The model under review builds one solid part; all positions refer to its coordinate system, in mm. Coordinates: 2 decimals unless noted, no trailing zeros. Order: outer loops, then holes, each group sorted by start corner. A loop starts at its lowest first (then second) coordinate and runs counter-clockwise, first axis right, second up. Notation, with made-up numbers: M -4.75,15.5 L 22.25,15.5 A34 ccw 22.25,48.5 Z; hole C 38,24.5 d2. An arc over 180 degrees is marked long. Answer as CSV lines item,"result". Start each with the question number.
Q1. Consider section A-A on x = 0. State how many separate pieces and enclosed holes the cut face has, and give its area (3 significant figures).
Q2. Wall thickness on L1, parallel to Z at x = 0, y = 1.75 (1 decimal); L2, parallel to Z at x = 10, y = 5.5; L3, parallel to Z at x = -1, y = 2.75: over which ranges is each line inside the solid? List them lowest first. Write a range as [from, to].
Q3. Consider section B-B on z = 81. Write out the cut boundary in (x, y), and give its area (3 significant figures).
Q4. For P1, Ø2, axis at x = 7, y = 5.5, coming from the -Z side; P2, Ø1, axis at y = 3, z = 38, coming from the -X side, all flat-tipped, find the tip position at first contact; note any pin that passes through.
Q5. Consider section C-C on x = -9.5. Write out the cut boundary in (y, z).
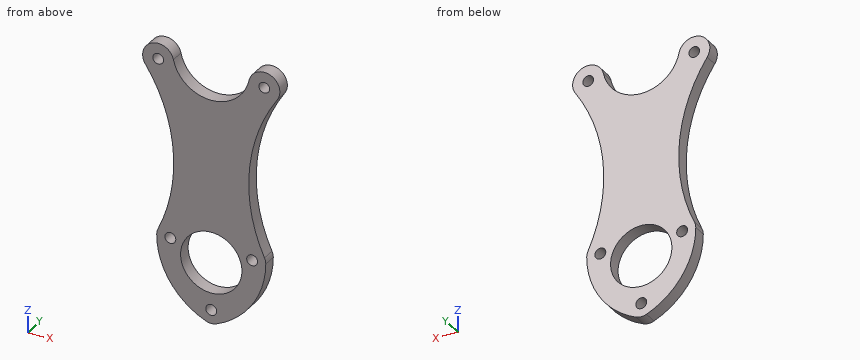
Autodesk Inventor part; units mm, degrees
ref_plane "YZ Plane" through (0, 0, 0) normal (1, 0, 0) x (0, 1, 0)
ref_plane "XZ Plane" through (0, 0, 0) normal (0, 1, 0) x (-1, 0, 0)
ref_plane "XY Plane" through (0, 0, 0) normal (0, 0, 1) x (1, 0, 0)
sketch "Sketch1" plane through (0, 0, 0) normal (0, 1, 0) x (-1, 0, 0)
  circle A0 centre (0, 0) radius 14.2875
  line L0 (143.7805, 15.875) -> (-143.7805, 15.875) construction
  line L1 (0, 0) -> (0, 15.875) construction
  line L2 (0, 15.875) -> (0, 88.9254) construction
  line L3 (24.6957, 88.9254) -> (-24.6957, 88.9254) construction
  line L4 (0, 113.6211) -> (0, 64.2297) construction
  circle A1 centre (24.6957, 88.9254) radius 2.4892
  circle A2 centre (-24.6957, 88.9254) radius 2.4892
  circle A3 centre (0, 64.2297) radius 2.4892 construction
  circle A4 centre (0, 113.6211) radius 2.4892 construction
  circle A5 centre (0, 0) radius 50.8 construction
  line L5 (143.7805, -34.925) -> (-143.7805, -34.925) construction
  line L6 (0, 0) -> (0, -34.925) construction
  circle A6 centre (19.05, 6.35) radius 2.54
  circle A7 centre (-19.05, 6.35) radius 2.54
  circle A8 centre (0, -22.225) radius 2.54
  line L7 (19.05, 6.35) -> (-19.05, 6.35) construction
  arc A9 (-2.4454, -28.0852) -> (2.4454, -28.0852) centre (0, -22.225) ccw
  arc A10 (-24.7931, 9.059) -> (-25.4, 6.3466) centre (-19.05, 6.35) ccw
  arc A11 (25.4, 6.3466) -> (24.7931, 9.059) centre (19.05, 6.35) ccw
  arc A12 (30.6963, 84.8535) -> (24.7931, 9.059) centre (94.1678, 41.783) ccw
  arc A13 (-24.7931, 9.059) -> (-30.6963, 84.8535) centre (-94.1678, 41.783) ccw
  arc A14 (2.4454, -28.0852) -> (25.4, 6.3466) centre (-11.9308, 6.3664) ccw
  arc A15 (-25.4, 6.3466) -> (-2.4454, -28.0852) centre (11.9308, 6.3664) ccw
  line L8 (12.3733, -7.1438) -> (20.6222, -11.9063) construction
  arc A16 (-17.6059, 90.4493) -> (-30.6963, 84.8535) centre (-24.6957, 88.9254) ccw
  arc A17 (30.6963, 84.8535) -> (17.6059, 90.4493) centre (24.6957, 88.9254) ccw
  arc A18 (-17.6059, 90.4493) -> (17.6059, 90.4493) centre (0, 94.2334) ccw
  line L9 (-17.4625, 41.783) -> (17.4625, 41.783) construction
  circle A19 centre (0, 88.9254) radius 12.7 construction
  point P0 (0, 6.35)
  dimension "d0" = 28.575
  dimension "d1" = 15.875
  dimension "d3" = 4.9784
  dimension "d4" = 88.9254
  dimension "d5" = 101.6
  dimension "d7" = 50.8
  dimension "d8" = 5.08
  dimension "d9" = 9.525
  dimension "d10" = 38.1
  dimension "d12" = 6.35
  dimension "d18" = 28.575
  dimension "d19" = 9.525
  dimension "d20" = 60
  dimension "d23" = 34.925
  dimension "d25" = 4.7625
  dimension "d26" = 34.925
  dimension "d27" = 25.4
extrude "Extrusion1" add sketch "Sketch1" along normal blind 6.35
properties material "Aluminum 6061"
Evaluation:
1,separate pieces,"3"
1,enclosed holes,"0"
1,area,"452 mm²"
2,L1,"z = [-28.6, -24.8], [-19.7, -14.3], [14.3, 76.2]"
2,L2,"z = [-23.84, -10.2], [10.2, 79.26]"
2,L3,"z = [-28.5, -24.56], [-19.89, -14.25], [14.25, 76.25]"
3,outline,"M -28.25,0 L -12.21,0 L -12.21,6.35 L -28.25,6.35 Z; M 12.21,0 L 28.25,0 L 28.25,6.35 L 12.21,6.35 Z"
3,area,"204 mm²"
4,P1,"stops at z = -26.38"
4,P2,"stops at x = -17.58"
5,outline,"M 0,-24.2 L 6.35,-24.2 L 6.35,-10.67 L 0,-10.67 Z; M 0,10.67 L 6.35,10.67 L 6.35,78.94 L 0,78.94 Z"
